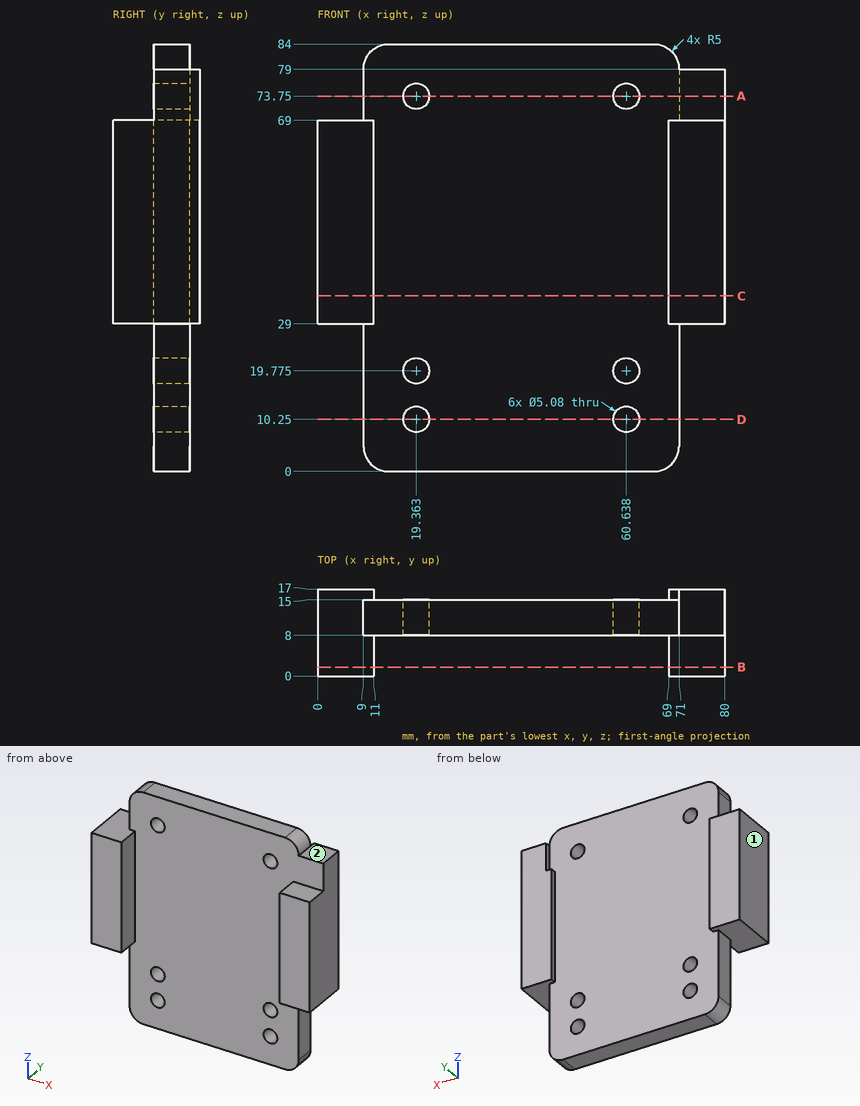
Drawing for the job (mm, zero at the part's lowest x, y, z). A direction names the side the tool comes from. Round coordinates to 2 decimals unless told otherwise and drop trailing zeros. Write each loop counter-clockwise with the first axis right and the second up, starting at its lowest first coordinate (ties: lowest second). Pieces come first, ordered by that corner, then holes. Notation, with made-up numbers: M -10,6 L -2,6 A25 ccw -2,39 Z; hole C 14,-30 d5. An arc over 180 degrees is marked long. One line per question, with ' | ' between items.
1. Cut at C-C on z = 34.5. Write the cut outline in (x, y), and give its area (3 significant figures).
Working result:
outline: M 0,0 L 11,0 L 11,8 L 69,8 L 69,0 L 80,0 L 80,17 L 69,17 L 69,15 L 11,15 L 11,17 L 0,17 Z | area: 780 mm2
2. Pin check, flat tips, straight feed: pin 1 Ø3.5 at (x, y) = (72, 10) entering from -Z (1 decimal); pin 2 Ø1.6 at (y, z) = (16, 73.5) entering from -X; pin 3 Ø2.5 at (x, y) = (77, 4.5) entering from +Z. Stop position of each tip, or through.
Working result:
pin 1: z = 2.4 | pin 2: x = 71 | pin 3: z = 69
3. Which spindle directions (+Z, -Z, +X, -X, +Y, -Y) get a long thin tool onto all of the face, cutting with end or side? Do the marked faces 1 and 2. Say none if no direction does.
Working result:
face 1: +Z, -Z, -X, +Y, -Y | face 2: +Z, +X, +Y, -Y
4. Probe L1, parallel to X at y = 9.75, z = 73.75; L2, parallel to X at y = 10.5, z = 10.25; L3, parallel to X at y = 2, z = 60. List the from-to ranges inside material, lowest first. Write a range as from..to.
Working result:
L1: 9..16.82, 21.9..58.1, 63.18..80 | L2: 9..16.82, 21.9..58.1, 63.18..71 | L3: 0..11, 69..80
5. Cut at D-D on z = 10.25. Write the cut outline in (x, y).
Working result:
outline: M 9,8 L 16.82,8 L 16.82,15 L 9,15 Z; M 21.9,8 L 58.1,8 L 58.1,15 L 21.9,15 Z; M 63.18,8 L 71,8 L 71,15 L 63.18,15 Z
6. Cut at A-A on z = 73.75. Write the cut outline in (x, y), and give its area (3 significant figures).
Working result:
outline: M 9,8 L 16.82,8 L 16.82,15 L 9,15 Z; M 21.9,8 L 58.1,8 L 58.1,15 L 21.9,15 Z; M 63.18,8 L 80,8 L 80,17 L 71,17 L 71,15 L 63.18,15 Z | area: 444 mm2
7. Cut at B-B on y = 1.75. Write the cut outline in (x, z), and give its area (3 significant figures).
Working result:
outline: M 0,29 L 11,29 L 11,69 L 0,69 Z; M 69,29 L 80,29 L 80,69 L 69,69 Z | area: 880 mm2
